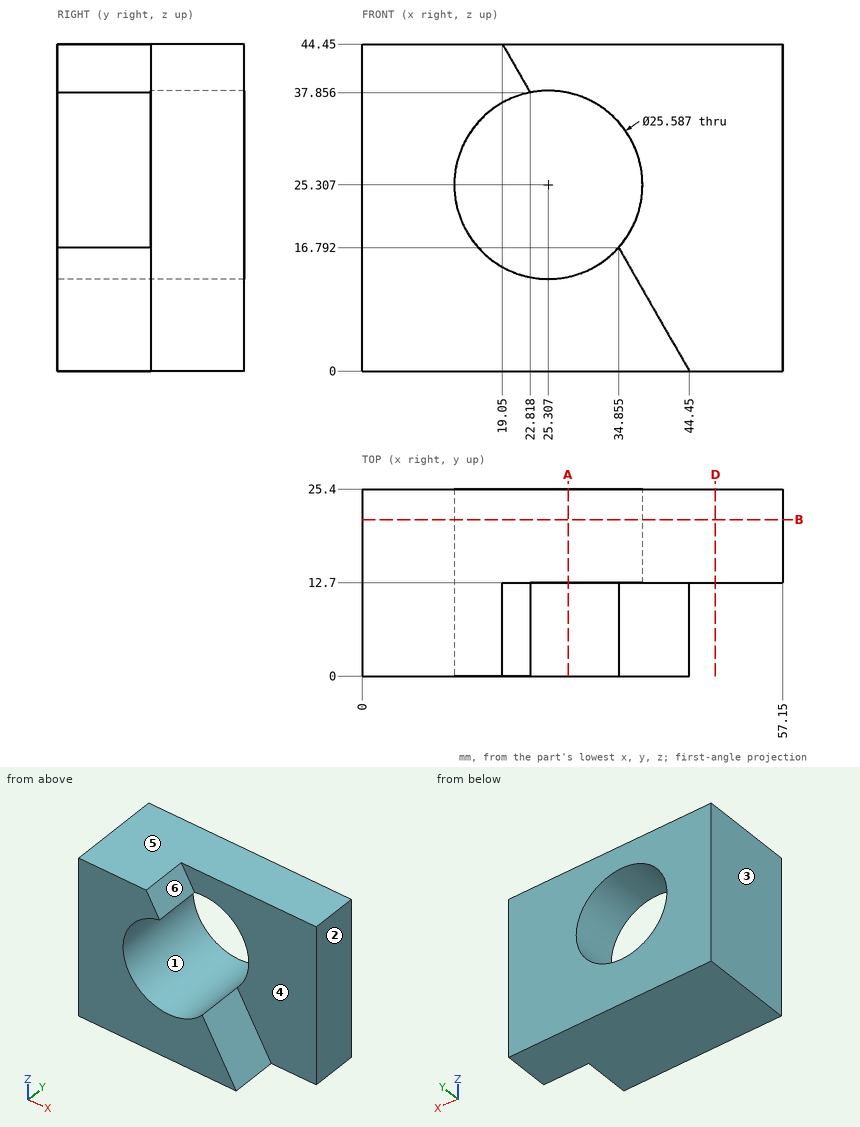
Part print with two shaded views. Sizes in mm from the minimum x, y, z corner. A direction names the side the tool comes from. Give positions to 0.01 mm unless a question says otherwise; leave off trailing zeros. Write each loop counter-clockwise with the first axis right and the second up, starting at its lowest first coordinate (ties: lowest second). Pieces come first, ordered by that corner, then holes.
1) Cut at D-D on x = 48. Write the cut outline in (y, z).
Resolved:
outline: (12.7, 0) - (25.4, 0) - (25.4, 44.45) - (12.7, 44.45) - close
2) Cut at A-A on x = 28. Write the cut outline in (y, z).
Resolved:
outline: (0, 0) - (25.4, 0) - (25.4, 12.8) - (0, 12.8) - close; (12.7, 37.81) - (25.4, 37.81) - (25.4, 44.45) - (12.7, 44.45) - close
3) Cut at B-B on y = 21.25. Write the cut outline in (x, z), then the cut area to 3 significant figures.
Resolved:
outline: (0, 0) - (57.15, 0) - (57.15, 44.45) - (0, 44.45) - close; hole circle Ø25.59 at (25.31, 25.31)
area: 2,030 mm2
4) Probe L1, parallel to Y at x = 54.5, z = 6.5; L2, parallel to Z at x = 25, y = 1.75; L3, parallel to X at y = 6, z = 39.5. List the from-to ranges inside material, lowest first.
Resolved:
L1: y = 12.7 to 25.4
L2: z = 0 to 12.52
L3: x = 0 to 21.88
5) Which spindle directions (+Z, -Z, +X, -X, +Y, -Y) get a long thin tool onto all of the face, cutting with end or side? Do the marked faces 5 and 6. Say none if no direction does.
Resolved:
face 5: +Z, +X, -X, +Y, -Y
face 6: +Z, +X, -Y
6) Two-plate mould, pull along X, no slides. Class the marked faces 1, 2, 3 and 4: released by +X, released by -X, zero draft, split by the parting line, or undercut.
Resolved:
face 1: undercut
face 2: released by +X
face 3: released by -X
face 4: zero draft
